```python
from build123d import *

# Parameters (mm, degrees)
SKETCH1_W           = 1200
SKETCH1_H           = 600
BOSS_EXTRUDE1_DEPTH = 25
SKETCH2_W           = 40
SKETCH2_H           = 40
BOSS_EXTRUDE2_DEPTH = 725
SKETCH3_W           = 1200
SKETCH3_H           = 600
BOSS_EXTRUDE3_DEPTH = 25
CHAMFER1_SIZE       = 2


with BuildPart() as part:
    # Sketch1 → Boss-Extrude1 (new body)
    with BuildSketch(Plane.XY):
        Rectangle(SKETCH1_W, SKETCH1_H)
    extrude(amount=BOSS_EXTRUDE1_DEPTH)

    # Sketch2 → Boss-Extrude2 (add)
    with BuildSketch(Plane.XY):
        with Locations((-560, -260)):
            Rectangle(SKETCH2_W, SKETCH2_H)
        with Locations((560, -260)):
            Rectangle(SKETCH2_W, SKETCH2_H)
        with Locations((560, 260)):
            Rectangle(SKETCH2_W, SKETCH2_H)
        with Locations((-560, 260)):
            Rectangle(SKETCH2_W, SKETCH2_H)
    extrude(amount=BOSS_EXTRUDE2_DEPTH)

    # Sketch3 → Boss-Extrude3 (add)
    with BuildSketch(Plane.XY.offset(725)):
        Rectangle(SKETCH3_W, SKETCH3_H)
    extrude(amount=BOSS_EXTRUDE3_DEPTH)

    # Chamfer1
    chamfer1_edges = [part.edges().sort_by_distance(p)[0] for p in [
        (600, -300, 737.5),
        (600, 300, 737.5),
        (-600, 300, 737.5),
        (-600, -300, 737.5),
    ]]
    chamfer(chamfer1_edges, length=CHAMFER1_SIZE)


solid = part.part
```
CAD build for the part. Positions are in the model's coordinates, mm. A direction names the side the tool comes from. Coordinates: 2 decimals unless noted, no trailing zeros. Loops run counter-clockwise (first coordinate to the right, second up) from the corner with the lowest first, then second, coordinate; pieces in that order, holes last. Notation, with made-up numbers: (46.25, -25.5) - (89.25, -25.5) arc R13 cw to (89.25, -14.5) - close; hole circle Ø3 at (37, 81). An arc over 180 degrees is marked (long way). Return JSON: item names as keys, results as strings.
1. 3-axis set-ups, long thin cutter, end or side, ignore diameter. For faces 1 (the flat face through (560, 280, 370)), 2 (the flat face through (-540, 260, 370)), 3 (the flat face through (580, 260, 370)), 4 (the flat face through (-560, -280, 370)): which of +Z, -Z, +X, -X, +Y, -Y reach the whole face in a straight line?
Result:
{"face 1": "+X, -X, +Y", "face 2": "+Y, -Y", "face 3": "+X, +Y, -Y", "face 4": "+X, -X, -Y"}
2. Mould opens along Z. For faces 5 (the flat face through (-8, 4, 725)), 6 (the flat face through (-8, 4, 750)), 7 (the flat face through (600, -4, 737)) say: released by +Z, released by -Z, zero draft, split by the parting line, or undercut.
Result:
{"face 5": "undercut", "face 6": "released by +Z", "face 7": "zero draft"}
3. Band-saw the part on A-A (x = 515). Give the cut face in (y, z).
Result:
{"outline": "(-300, 0) - (300, 0) - (300, 25) - (-300, 25) - close; (-300, 725) - (300, 725) - (300, 750) - (-300, 750) - close"}
4. Band-saw the part on B-B (y = 112.5). Give the cut face in (x, z), and give its area (3 significant figures).
Result:
{"outline": "(-600, 0) - (600, 0) - (600, 25) - (-600, 25) - close; (-600, 725) - (600, 725) - (600, 750) - (-600, 750) - close", "area": "60,000 mm2"}
5. Drop flat-ended pins along their axis: pin 1 (20 mm diameter, centred on y = 262, z = 261.5, fed in from +X); pin 2 (20 mm diameter, centred on y = 259, z = 387.5, fed in from -X); pin 3 (20 mm diameter, centred on x = -570, z = 357, fed in from +Y). Give the stop position or say it passes through.
Result:
{"pin 1": "stops at x = 580", "pin 2": "stops at x = -580", "pin 3": "stops at y = 280"}
6. Band-saw the part on C-C (z = 496). Give the cut face in (x, y), and give its area (3 significant figures).
Result:
{"outline": "(-580, -280) - (-540, -280) - (-540, -240) - (-580, -240) - close; (-580, 240) - (-540, 240) - (-540, 280) - (-580, 280) - close; (540, -280) - (580, -280) - (580, -240) - (540, -240) - close; (540, 240) - (580, 240) - (580, 280) - (540, 280) - close", "area": "6,400 mm2"}
7. Probe L1, parallel to Z at x = 247, y = 156.5. List the from-to ranges inside material, lowest first. Write a range as from..to.
Result:
{"L1": "z = 0..25, 725..750"}
